Verification items for the finished model (mm, model axes). A direction names the side the tool comes from. Round coordinates to 2 decimals unless told otherwise and drop trailing zeros. Loops run counter-clockwise (first coordinate to the right, second up) from the corner with the lowest first, then second, coordinate; pieces in that order, holes last.
from build123d import *

# Parameters (mm, degrees)
SKETCH_1_R          = 60
EXTRUDE_1_DEPTH     = 15
SKETCH_2_R          = 6
CUT_EXTRUDE_1_DEPTH = 87.168439698
SKETCH_3_R          = 11
CUT_EXTRUDE_2_DEPTH = 8
SKETCH_4_R          = 6.5
CUT_EXTRUDE_3_DEPTH = 10
SKETCH_5_R          = 3.3
CUT_EXTRUDE_4_DEPTH = 10


with BuildPart() as part:
    # 草图1 → 凸台-拉伸1 (new body)
    with BuildSketch(Plane.XY):
        Circle(SKETCH_1_R)
    extrude(amount=EXTRUDE_1_DEPTH)

    # 草图2 → 切除-拉伸1 (cut, through all)
    with BuildSketch(Plane(origin=(0, 0, 0), x_dir=(-1, 0, 0), z_dir=(0, 0, -1))):
        with Locations((-35, 0)):
            Circle(SKETCH_2_R)
        with Locations((35, 0)):
            Circle(SKETCH_2_R)
    extrude(amount=-CUT_EXTRUDE_1_DEPTH, mode=Mode.SUBTRACT)

    # 草图3 → 切除-拉伸2 (cut)
    with BuildSketch(Plane(origin=(0, 0, 0), x_dir=(-1, 0, 0), z_dir=(0, 0, -1))):
        Circle(SKETCH_3_R)
    extrude(amount=-CUT_EXTRUDE_2_DEPTH, mode=Mode.SUBTRACT)

    # 草图4 → 切除-拉伸3 (cut)
    with BuildSketch(Plane(origin=(0, 0, 8), x_dir=(-1, 0, 0), z_dir=(0, 0, -1))):
        Circle(SKETCH_4_R)
    extrude(amount=-CUT_EXTRUDE_3_DEPTH, mode=Mode.SUBTRACT)

    # 草图5 → 切除-拉伸4 (cut)
    with BuildSketch(Plane.XY.offset(15)):
        with Locations((40, 15)):
            Circle(SKETCH_5_R)
        with Locations((40, -15)):
            Circle(SKETCH_5_R)
        with Locations((-40, -15)):
            Circle(SKETCH_5_R)
        with Locations((-40, 15)):
            Circle(SKETCH_5_R)
    extrude(amount=-CUT_EXTRUDE_4_DEPTH, mode=Mode.SUBTRACT)


solid = part.part
1. Section check C-C (x = 0). Enter the section's corners in (y, z).
2. Gauge pin test, flat ends, axial feed: P1, Ø5, axis at x = -20.5, z = 7, coming from the +Y side; P2, Ø3.5, axis at x = 41, y = 16, coming from the +Z side; P3, Ø1.5, axis at x = 31.5, z = 11, coming from the +Y side. Record the tip position at first contact, or that the pin passes through.
3. Section check D-D (z = 3.5). Enter the section's corners in (x, y), then the cut area to 3 significant figures.
4. Release check for a two-part mould opening along Y. For faces 4 (the face through (-5, -5, 8)), 5 (the face through (-59.94, 2.64, 7.4)), 6 (the face through (12, 1, 0)) record: released by +Y, released by -Y, zero draft, split by the parting line, or undercut.
5. Scan lines: L1, parallel to Y at x = 0, z = 11; L2, parallel to Y at x = 40, z = 1; L3, parallel to X at y = -13.5, z = 14. Record each from-to range of solid material in increasing order.
6. Tool access check on faces 1 (the face through (2.38, -10.74, 3.94)), 2 (the face through (40, 15, 5)), 3 (the face through (12, 1, 15)). Record the directions out of +Z, -Z, +X, -X, +Y, -Y that give a thin tool (end or side, any length) a straight path to the whole face; none if there is none.
7. Section check B-B (z = 11.75). Enter the section's corners in (x, y).
8. Section check A-A (y = 0). Enter the section's corners in (x, z), then the cut area to 3 significant figures.
Taken from the geometry:
1. outline: (-60, 0) - (-11, 0) - (-11, 8) - (-6.5, 8) - (-6.5, 15) - (-60, 15) - close; (6.5, 8) - (11, 8) - (11, 0) - (60, 0) - (60, 15) - (6.5, 15) - close
2. P1: stops at y = 57.24
2. P2: stops at z = 5
2. P3: stops at y = 51.52
3. outline: circle Ø120 at (0, 0); hole circle Ø12 at (-35, 0); hole circle Ø22 at (0, 0); hole circle Ø12 at (35, 0)
3. area: 10,700 mm2
4. face 4: undercut
4. face 5: split by the parting line
4. face 6: zero draft
5. L1: y = -60 to -6.5, 6.5 to 60
5. L2: y = -44.72 to -3.32, 3.32 to 44.72
5. L3: x = -58.46 to -42.94, -37.06 to 37.06, 42.94 to 58.46
6. face 1: -Z
6. face 2: +Z
6. face 3: +Z, +X, -X, +Y, -Y
7. outline: circle Ø120 at (0, 0); hole circle Ø6.6 at (-40, -15); hole circle Ø6.6 at (-40, 15); hole circle Ø12 at (-35, 0); hole circle Ø13 at (0, 0); hole circle Ø12 at (35, 0); hole circle Ø6.6 at (40, -15); hole circle Ø6.6 at (40, 15)
8. outline: (-60, 0) - (-41, 0) - (-41, 15) - (-60, 15) - close; (-29, 0) - (-11, 0) - (-11, 8) - (-6.5, 8) - (-6.5, 15) - (-29, 15) - close; (6.5, 8) - (11, 8) - (11, 0) - (29, 0) - (29, 15) - (6.5, 15) - close; (41, 0) - (60, 0) - (60, 15) - (41, 15) - close
8. area: 1,170 mm2
